Build history of the part. All positions in model axes, mm. Face numbers are marked on the shaded views. A direction names the side the tool comes from. Coordinates: 2 decimals unless noted, no trailing zeros. Order: outer loops, then holes, each group sorted by start corner. A loop starts at its lowest first (then second) coordinate and runs counter-clockwise, first axis right, second up. Notation, with made-up numbers: M 61.5,24.25 L 102.5,24.25 A24 ccw 102.5,41.25 Z; hole C -21.5,-18 d1. An arc over 180 degrees is marked long. Write item = value, one per line. Start each with the question number.
Q1. Band-saw the part on D-D on x = 6.25. Write the cut outline in (y, z), plus the area to 3 significant figures.
Q2. 3-axis set-ups, long thin cutter, end or side, ignore diameter. For the marked faces 4, 5 and 6: which of +Z, -Z, +X, -X, +Y, -Y reach the whole face in a straight line?
Q3. Band-saw the part on B-B on z = -2.25. Write the cut outline in (x, y).
Q4. Drill centre lines: probe 1 along Y at (x, z) = (0, -5); probe 2 along Z at (x, y) = (5.75, 0.25); probe 3 along X at (y, z) = (0.25, -6). Where is each one in solid material? Low to high.
Q5. Band-saw the part on C-C on y = 0.75. Write the cut outline in (x, z).
Q6. Band-saw the part on A-A on x = 0. Write the cut outline in (y, z).
Q7. Pin check, flat tips, straight feed: P1, Ø3, axis at y = 5.5, z = -1.5, coming from the -X side; P2, Ø8.5, axis at x = -1.5, y = 3.5, coming from the +Z side; P3, Ø2, axis at x = -1, y = -1, coming from the -Z side; P4, Ø2, axis at x = 1, y = -1.5, coming from the +Z side. Stop position of each tip, or through.
Q8. Pull direction Y, two halves, no side cores. Call the marked faces 1, 2 and 3: released by +Y, released by -Y, zero draft, split by the parting line, or undercut.
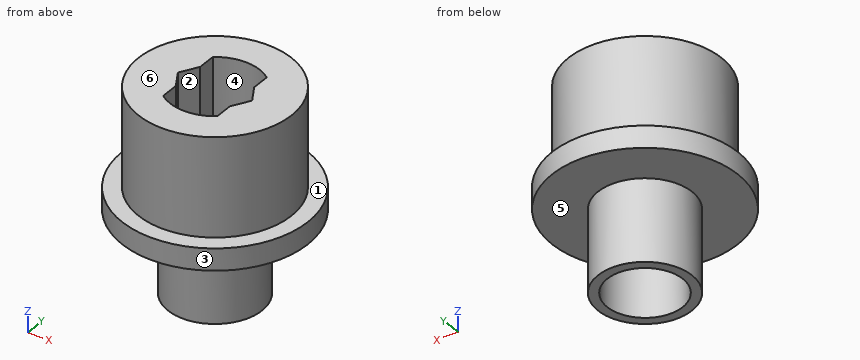
```python
from build123d import *

# Parameters (mm, degrees)
SKETCH1_R               = 7
SKETCH1_R_2             = 4.1
BOSS_EXTRUDE1_DEPTH     = 9
SKETCH5_R               = 8.5
BOSS_EXTRUDE3_DEPTH     = 2
CUT_EXTRUDE4_DEPTH      = 16.016657418
SKETCH10_R              = 4.3
BOSS_EXTRUDE4_DEPTH     = 7.5
CUT_EXTRUDE8_DEPTH      = 17.294170737
CUT_EXTRUDE8_DEPTH_BACK = 1
SKETCH6_R               = 3.45


with BuildPart() as part:
    # Sketch1 → Boss-Extrude1 (new body)
    # profile 1 of 3: a face of its own
    with BuildSketch(Plane.XY):
        Circle(SKETCH1_R)
        Circle(SKETCH1_R_2, mode=Mode.SUBTRACT)
    # profile 2 of 3: a face of its own
    with BuildSketch(Plane.XY):
        with BuildLine():
            Line((-2.475, -3.268696223), (-2.475, 3.268696223))
            ThreePointArc((-2.475, 3.268696223), (-4.1, 0), (-2.475, -3.268696223))
        make_face()
    # profile 3 of 3: a face of its own
    with BuildSketch(Plane.XY):
        with BuildLine():
            ThreePointArc((4.1, 0), (3.671341717, 1.825171225), (2.475, 3.268696223))
            Line((2.475, 3.268696223), (2.475, -3.268696223))
            ThreePointArc((2.475, -3.268696223), (3.671341717, -1.825171225), (4.1, 0))
        make_face()
    extrude(amount=BOSS_EXTRUDE1_DEPTH)

    # Sketch5 → Boss-Extrude3 (add)
    with BuildSketch(Plane(origin=(0, 0, 0), x_dir=(-1, 0, 0), z_dir=(0, 0, -1))):
        Circle(SKETCH5_R)
    extrude(amount=BOSS_EXTRUDE3_DEPTH)

    # Sketch9 → Cut-Extrude4 (cut, through all)
    with BuildSketch(Plane.XY):
        Polygon((-3.4, 0), (-1.7, -2.944486373), (1.7, -2.944486373), (3.4, 0), (1.7, 2.944486373), (-1.7, 2.944486373), align=None)
    extrude(amount=CUT_EXTRUDE4_DEPTH, mode=Mode.SUBTRACT)

    # Sketch10 → Boss-Extrude4 (add)
    with BuildSketch(Plane(origin=(0, 0, -2), x_dir=(-1, 0, 0), z_dir=(0, 0, -1))):
        Circle(SKETCH10_R)
    extrude(amount=BOSS_EXTRUDE4_DEPTH)

    # Sketch6 → Cut-Extrude8 (cut, two sides: drawn at the far end of the back side and taken through both)
    with BuildSketch(Plane(origin=(0, 0, -2), x_dir=(-1, 0, 0), z_dir=(0, 0, -1)).offset(-CUT_EXTRUDE8_DEPTH_BACK)):
        Circle(SKETCH6_R)
    extrude(amount=CUT_EXTRUDE8_DEPTH + CUT_EXTRUDE8_DEPTH_BACK, mode=Mode.SUBTRACT)


solid = part.part
```
Recorded:
q1.outline = M -5.76,-2 L 5.76,-2 L 5.76,0 L 3.15,0 L 3.15,9 L -3.15,9 L -3.15,0 L -5.76,0 Z
q1.area = 79.8 mm2
q2.face_4 = +Z
q2.face_5 = -Z
q2.face_6 = +Z, +X, -X, +Y, -Y
q3.outline = C 0,0 d8.6; hole C 0,0 d6.9
q4.probe_1 = -4.3 to -3.45, 3.45 to 4.3
q4.probe_2 = -2 to 9
q4.probe_3 = -4.29 to -3.44, 3.44 to 4.29
q5.outline = M -8.47,-2 L -4.23,-2 L -4.23,-9.5 L -3.37,-9.5 L -3.37,-1 L 3.37,-1 L 3.37,-9.5 L 4.23,-9.5 L 4.23,-2 L 8.47,-2 L 8.47,0 L 6.96,0 L 6.96,9 L 2.97,9 L 2.97,0 L -2.97,0 L -2.97,9 L -6.96,9 L -6.96,0 L -8.47,0 Z
q6.outline = M -8.5,-2 L -4.3,-2 L -4.3,-9.5 L -3.45,-9.5 L -3.45,-1 L 3.45,-1 L 3.45,-9.5 L 4.3,-9.5 L 4.3,-2 L 8.5,-2 L 8.5,0 L 7,0 L 7,9 L 4.1,9 L 4.1,0 L -4.1,0 L -4.1,9 L -7,9 L -7,0 L -8.5,0 Z
q7.P1 = -7.5
q7.P2 = 9
q7.P3 = -1
q7.P4 = 0
q8.face_1 = zero draft
q8.face_2 = undercut
q8.face_3 = split by the parting line
